```python
from build123d import *

# Parameters (mm, degrees)
EXTRUDE_1_DEPTH     = 45
SKETCH_2_R          = 1.6
CUT_EXTRUDE_1_DEPTH = 35
FILLET_1_R          = 5
SKETCH_3_R          = 15
EXTRUDE_2_DEPTH     = 10
SKETCH_7_R          = 22.5
EXTRUDE_3_DEPTH     = 5
FILLET_2_R          = 10


with BuildPart() as part:
    # ｽｹｯﾁ1 → ﾎﾞｽ - 押し出し1 (new body)
    with BuildSketch(Plane.XY):
        Polygon((0, 30), (0, 0), (50, 0), (50, 2), (2, 2), (2, 30), align=None)
    extrude(amount=EXTRUDE_1_DEPTH)

    # ｽｹｯﾁ2 → ｶｯﾄ - 押し出し1 (cut)
    with BuildSketch(Plane.ZY):
        with Locations((40, 25)):
            Circle(SKETCH_2_R)
        with Locations((5, 25)):
            Circle(SKETCH_2_R)
    extrude(amount=-CUT_EXTRUDE_1_DEPTH, mode=Mode.SUBTRACT)

    # ﾌｨﾚｯﾄ1
    fillet_1_edges = [part.edges().sort_by_distance(p)[0] for p in [
        (50, 1, 45),
        (50, 1, 0),
    ]]
    fillet(fillet_1_edges, radius=FILLET_1_R)

    # ｽｹｯﾁ3 → ﾎﾞｽ - 押し出し2 (add)
    with BuildSketch(Plane.XZ):
        with Locations(Location((25, 22.5, 0), (0, 0, 90))):
            Circle(SKETCH_3_R)
    extrude(amount=EXTRUDE_2_DEPTH)

    # ｽｹｯﾁ7 → ﾎﾞｽ - 押し出し3 (add)
    with BuildSketch(Plane(origin=(0, -10, 0), x_dir=(-1, 0, 0), z_dir=(0, -1, 0))):
        with Locations(Location((-25, -22.5, 0), (0, 0, 90))):
            Circle(SKETCH_7_R)
    extrude(amount=EXTRUDE_3_DEPTH)

    # ﾌｨﾚｯﾄ2
    # the kernel refuses this fillet: 10 mm, written as the material it takes off along each edge
    with BuildSketch(Plane(origin=(25, -15, 22.5), x_dir=(0, 0, -1), z_dir=(-1, 0, 0))) as fillet_2_piece_1:
        with BuildLine():
            CenterArc((13.839745962, -10), FILLET_2_R, 30, 60)
            Line((13.839745962, 0), (13.839745962, 0.2))
            Line((13.839745962, 0.2), (22.5, 0.2))
            Line((22.5, 0.2), (22.7, 0))
            ThreePointArc((22.7, 0), (22.7, -2.5), (22.673205081, -4.9))
            Line((22.673205081, -4.9), (22.5, -5))
        make_face()
    revolve(axis=Axis((25, -15, 22.5), (0, -1, 0)), mode=Mode.SUBTRACT)


solid = part.part
```
Here's how the part is built. I have some questions about the finished solid (model axes, mm). A direction names the side the tool comes from. Give positions to 0.01 mm unless a question says otherwise; leave off trailing zeros. Loops run counter-clockwise (first coordinate to the right, second up) from the corner with the lowest first, then second, coordinate; pieces in that order, holes last. Notation, with made-up numbers: (-5.75, 13) -> (15.25, 13) arc R15 cw to (15.25, 21) -> close; hole circle Ø1 at (-32.75, 43.25). An arc over 180 degrees is marked (long way). Use one line per item in the form item = value. Start each with the question number.
1) Imagine slicing it at C-C (x = 25). Please give me the cut outline in (y, z).
2) Imagine slicing it at A-A (y = 25). Please give me the cut outline in (x, z).
3) Which directions (+Z, -Z, +X, -X, +Y, -Y) give clear straight access to the entire face, cutting with the end or side of a thin tool? Please do faces 1 (the face through (0, 15, 22)), 2 (the face through (26, 2, 22)), 3 (the face through (39.643, -4.93, 19.248)).
4) Thinking about a two-plate mould opening in Y: for faces 4 (the face through (1, 30, 22)), 5 (the face through (48, 1, 44)), 6 (the face through (14, 0, 12)), which applies, +Y half, -Y half, draft (parallel to the pull), parting line (faces both ways), or undercut?
5) Imagine slicing it at B-B (z = 22.5). Please give me the cut outline in (x, y).
6) Imagine slicing it at D-D (y = 16). Please give me the cut outline in (x, z), then the cut area to 3 significant figures.
7) For P1, Ø13.5, axis at x = 19.5, z = 24, coming from the +Y side; P2, Ø2, axis at x = 11, z = 9, coming from the -Y side; P3, Ø4, axis at y = 25, z = 5, coming from the +X side, each with a flat end and sliding along its axis, tell me the tip position at first contact or that it passes through.
8) Please list where these lines run through material, in increasing order: line 1 along Y through (x, z) = (1.5, 40); line 2 along X through (y, z) = (15, 6); line 3 along Y through (x, z) = (39, 8.5).
Check values:
q1.outline = (-15, 8.66) arc R10 ccw to (-10, 0) -> (-10, 7.5) -> (0, 7.5) -> (0, 0) -> (2, 0) -> (2, 45) -> (0, 45) -> (0, 37.5) -> (-10, 37.5) -> (-10, 45) arc R10 ccw to (-15, 36.34) -> close
q2.outline = (0, 0) -> (2, 0) -> (2, 3.4) -> (0, 3.4) -> close; (0, 6.6) -> (2, 6.6) -> (2, 38.4) -> (0, 38.4) -> close; (0, 41.6) -> (2, 41.6) -> (2, 45) -> (0, 45) -> close
q3.face_1 = +Z, -Z, -X, +Y, -Y
q3.face_2 = +Z, -Z, +X, +Y
q3.face_3 = none
q4.face_4 = +Y half
q4.face_5 = draft
q4.face_6 = undercut
q5.outline = (0, 0) -> (10, 0) -> (10, -10) -> (2.5, -10) arc R10 ccw to (11.16, -15) -> (38.84, -15) arc R10 ccw to (47.5, -10) -> (40, -10) -> (40, 0) -> (50, 0) -> (50, 2) -> (2, 2) -> (2, 30) -> (0, 30) -> close
q6.outline = (0, 0) -> (2, 0) -> (2, 45) -> (0, 45) -> close
q6.area = 90.0 mm^2
q7.P1 = 2
q7.P2 = -13.87
q7.P3 = 2
q8.line_1 = 0 to 23.4, 26.6 to 30
q8.line_2 = 0 to 2
q8.line_3 = -13.03 to -10, 0 to 2
